Part model, mm, in its own coordinate system. A direction names the side the tool comes from. Coordinates: 2 decimals unless noted, no trailing zeros. Loops run counter-clockwise (first coordinate to the right, second up) from the corner with the lowest first, then second, coordinate; pieces in that order, holes last. Notation, with made-up numbers: (45, -25) - (83, -25) arc R33 cw to (83, 13) - close; hole circle Ø5 at (87.25, -34). An arc over 180 degrees is marked (long way). Use a Markdown table: item, result. Add a question column.
1. 3-axis set-ups, long thin cutter, end or side, ignore diameter. For faces 4 (the cylindrical face through (11.18, 6.06, 4.63)), 5 (the cylindrical face through (-8.098, 1.014, -4.926)): which of +Z, -Z, +X, -X, +Y, -Y reach the whole face in a straight line?
2. Band-saw the part on B-B, the plane z = 8.5. Give the cut face in (x, y), plus the area to 3 significant figures.
3. Wall check: probe 1 along Z at (x, y) = (0, 4.75); probe 2 along Z at (x, y) = (0, 1.25). Give the ranges that are in metal, low to high. Write a range as [from, to].
4. Pull direction X, two halves, no side cores. Call faces 1 (the flat face through (9, 10, 9)), 2 (the cylindrical face through (-0.13, 1.01, 7.51)), 3 (the cylindrical face through (-10.316, 4.93, 7.91)): pulls with the +X half, pulls with the -X half, needs draft (parallel to the pull), parting line crosses it, or undercut.
5. Band-saw the part on C-C, the plane z = 0. Give the cut face in (x, y).
6. Drop flat-ended pins along their axis: pin 1 (1 mm diameter, centred on x = 9, y = 4.5, fed in from -Z); pin 2 (2.5 mm diameter, centred on x = -7.36, z = -4.25, fed in from -Y); pin 3 (3 mm diameter, centred on x = 7.36, z = -4.25, fed in from +Y); pin 4 (1.8 mm diameter, centred on x = 0, z = 8.5, fed in from -Y). Give the stop position or say it passes through.
7. Band-saw the part on A-A, the plane x = 0. Give the cut face in (y, z), plus the area to 3 significant figures.
8. Band-saw the part on D-D, the plane y = 1. Give the cut face in (x, z).
from build123d import *

# Parameters (mm, degrees)
SKETCH2_R           = 13
BOSS_EXTRUDE2_DEPTH = 10
SKETCH5_R           = 12.1
CUT_EXTRUDE2_DEPTH  = 8
SKETCH6_R           = 1
CUT_EXTRUDE3_DEPTH  = 8


with BuildPart() as part:
    # Sketch2 → Boss-Extrude2 (new body)
    with BuildSketch(Plane(origin=(0, 0, 0), x_dir=(1, 0, 0), z_dir=(0, 1, 0))):
        Circle(SKETCH2_R)
    extrude(amount=BOSS_EXTRUDE2_DEPTH)

    # Sketch5 → Cut-Extrude2 (cut)
    with BuildSketch(Plane(origin=(0, 10, 0), x_dir=(1, 0, 0), z_dir=(0, 1, 0))):
        Circle(SKETCH5_R)
    extrude(amount=-CUT_EXTRUDE2_DEPTH, mode=Mode.SUBTRACT)

    # Sketch6 → Cut-Extrude3 (cut)
    with BuildSketch(Plane(origin=(0, 2, 0), x_dir=(1, 0, 0), z_dir=(0, 1, 0))):
        with Locations((0, -8.5)):
            Circle(SKETCH6_R)
        with Locations((-7.361215932, 4.25)):
            Circle(SKETCH6_R)
        with Locations((7.361215932, 4.25)):
            Circle(SKETCH6_R)
    extrude(amount=-CUT_EXTRUDE3_DEPTH, mode=Mode.SUBTRACT)


solid = part.part
Geometry check:
| question | item | result |
|---|---|---|
| 1 | face 4 | +Y |
| 1 | face 5 | +Y, -Y |
| 2 | outline | (-9.84, 0) - (-1, 0) - (-1, 2) - (-8.61, 2) - (-8.61, 10) - (-9.84, 10) - close; (1, 0) - (9.84, 0) - (9.84, 10) - (8.61, 10) - (8.61, 2) - (1, 2) - close |
| 2 | area | 54.9 mm^2 |
| 3 | probe 1 | z = [-13, -12.1], [12.1, 13] |
| 3 | probe 2 | z = [-13, 7.5], [9.5, 13] |
| 4 | face 1 | needs draft |
| 4 | face 2 | undercut |
| 4 | face 3 | parting line crosses it |
| 5 | outline | (-13, 0) - (13, 0) - (13, 10) - (12.1, 10) - (12.1, 2) - (-12.1, 2) - (-12.1, 10) - (-13, 10) - close |
| 6 | pin 1 | stops at z = -9.84 |
| 6 | pin 2 | stops at y = 0 |
| 6 | pin 3 | stops at y = 2 |
| 6 | pin 4 | passes through |
| 7 | outline | (0, -13) - (10, -13) - (10, -12.1) - (2, -12.1) - (2, 7.5) - (0, 7.5) - close; (0, 9.5) - (2, 9.5) - (2, 12.1) - (10, 12.1) - (10, 13) - (0, 13) - close |
| 7 | area | 62.4 mm^2 |
| 8 | outline | circle Ø26 at (0, 0); hole circle Ø2 at (-7.36, -4.25); hole circle Ø2 at (0, 8.5); hole circle Ø2 at (7.36, -4.25) |
